```python
from build123d import *

# Parameters (mm, degrees)
SKETCH1_R           = 42.2275
SKETCH1_R_2         = 39.6875
BOSS_EXTRUDE1_DEPTH = 259.08
SKETCH2_W           = 4.7625
SKETCH2_H           = 254
CUT_EXTRUDE1_DEPTH  = 266.873597622
CIRPATTERN1_COUNT   = 3


with BuildPart() as part:
    # Sketch1 → Boss-Extrude1 (new body)
    with BuildSketch(Plane.YZ):
        with Locations(Location((0, 0, 0), (0, 0, 270))):
            Circle(SKETCH1_R)
        with Locations(Location((0, 0, 0), (0, 0, 270))):
            Circle(SKETCH1_R_2, mode=Mode.SUBTRACT)
    extrude(amount=BOSS_EXTRUDE1_DEPTH)

    # Sketch2 → Cut-Extrude1 (cut, through all)
    with BuildSketch(Plane(origin=(0, 0, 0), x_dir=(0, 1, 0), z_dir=(0, 0, 1))):
        with Locations((0, -132.08)):
            Rectangle(SKETCH2_W, SKETCH2_H)
    cut_extrude1 = extrude(amount=CUT_EXTRUDE1_DEPTH, mode=Mode.SUBTRACT)

    # CirPattern1: Cut-Extrude1 ×3 about axis
    cirpattern1_axis = Axis((0, 0, 0), (1, 0, 0))
    for i in range(1, CIRPATTERN1_COUNT):
        add(cut_extrude1.rotate(cirpattern1_axis, i * 360 / CIRPATTERN1_COUNT), mode=Mode.SUBTRACT)


solid = part.part
```
Model file for the job. Use its own axes, mm. A direction names the side the tool comes from. Coordinates: 2 decimals unless noted, no trailing zeros. Order: outer loops, then holes, each group sorted by start corner. A loop starts at its lowest first (then second) coordinate and runs counter-clockwise, first axis right, second up. Notation, with made-up numbers: (86, 18.5) -> (145, 18.5) arc R35 cw to (145, 54.5) -> close; hole circle Ø7 at (-30, 57). An arc over 180 degrees is marked (long way). Answer as a JSON object with one key per item and string values. Group by question number.
1) Pull direction Z, two halves, no side cores. Call faces 1 (the face through (127.726, 41.868, 5.497)), 2 (the face through (127.726, 11.921, -37.855)), 3 (the face through (5.08, -35, -20)), 4 (the face through (0, -12, 38)): +Z half, -Z half, draft (parallel to the pull), parting line (faces both ways), or undercut.
2) Flat gauge pins, fed straight in: pin 1 (3 mm diameter, centred on x = 52.5, y = 30, fed in from -Z); pin 2 (1 mm diameter, centred on x = 151, y = -11.5, fed in from -Z); pin 3 (5 mm diameter, centred on x = 126.5, z = 17, fed in from -Y). Where does each tip first touch, or does it go through?
3) Drill centre lines: L1, parallel to Y at x = 179.5, z = 0; L2, parallel to Z at x = 79, y = 0; L3, parallel to Z at x = 22, y = 29. Where is each one in solid material? Low to high.
4) Cut at B-B, the plane z = -10.5. Write the cut outline in (x, y), then the cut area to 3 significant figures.
5) Which spindle directions (+Z, -Z, +X, -X, +Y, -Y) get a long thin tool onto all of the face, cutting with end or side? Do faces 5 (the face through (5.08, 35, -20)), 6 (the face through (259.08, -34, 21)). Say none if no direction does.
6) Cut at C-C, the plane x = 39.5. Write the cut outline in (y, z) (1 decimal).
7) Cut at A-A, the plane y = 0. Write the cut outline in (x, z), then the cut area to 3 significant figures.
Check values:
{
 "1": {"face 1": "parting line", "face 2": "undercut", "face 3": "undercut", "face 4": "draft"},
 "2": {"pin 1": "stops at z = -31.16", "pin 2": "stops at z = -40.77", "pin 3": "stops at y = -39.66"},
 "3": {"L1": "y = -42.23 to -39.69, 39.69 to 42.23", "L2": "z = -42.23 to -39.69", "L3": "z = -30.69 to -27.09, 27.09 to 30.69"},
 "4": {"outline": "(0, -40.9) -> (259.08, -40.9) -> (259.08, -38.27) -> (0, -38.27) -> close; (0, 38.27) -> (259.08, 38.27) -> (259.08, 40.9) -> (0, 40.9) -> close", "area": "1,360 mm²"},
 "5": {"face 5": "+X", "face 6": "+Z, -Z, +X, +Y, -Y"},
 "6": {"outline": "(-37.7, -19) -> (-35.5, -17.7) arc R39.7 cw to (-2.4, 39.6) -> (-2.4, 42.2) arc R42.2 ccw to start; (-35.3, -23.1) arc R42.2 ccw to (35.3, -23.1) -> (33.1, -21.9) arc R39.7 cw to (-33.1, -21.9) -> close; (2.4, 39.6) arc R39.7 cw to (35.5, -17.7) -> (37.7, -19) arc R42.2 ccw to (2.4, 42.2) -> close"},
 "7": {"outline": "(0, -42.23) -> (259.08, -42.23) -> (259.08, -39.69) -> (0, -39.69) -> close; (0, 39.69) -> (5.08, 39.69) -> (5.08, 42.23) -> (0, 42.23) -> close", "area": "671 mm²"}
}
